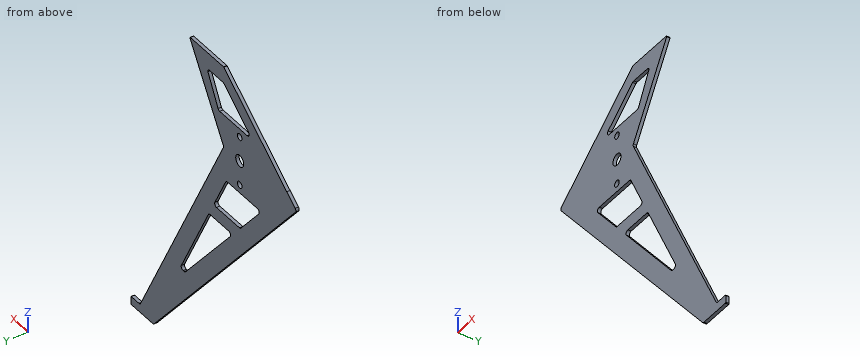
from build123d import *

# Parameters (mm, degrees)
F0_R     = 1.27
F0_R_2   = 2.2225
F1_DEPTH = 1.27


with BuildPart() as f1:
    # F0 (on Front) → F1 (new body)
    with BuildSketch(Plane.XZ):
        with BuildLine():
            Line((14.791388, 63.5), (-3.722544, 63.5))
            ThreePointArc((-3.722544, 63.5), (-3.805236, 63.486163), (-3.878918, 63.446158))
            Line((-3.878918, 63.446158), (-38.962514, 36.037098))
            Line((-38.962514, 36.037098), (-43.621762, 32.397061))
            ThreePointArc((-43.621762, 32.397061), (-44.006646, 31.703164), (-43.775246, 30.944163))
            Line((-43.775246, 30.944163), (-41.186804, 27.852871))
            Line((-41.186804, 27.852871), (35.001432, -63.136264))
            ThreePointArc((35.001432, -63.136264), (35.350553, -63.404586), (35.78041, -63.5))
            Line((35.78041, -63.5), (44.45, -63.5))
            Line((44.45, -63.5), (47.752, -63.5))
            ThreePointArc((47.752, -63.5), (47.931605, -63.425605), (48.006, -63.246))
            Line((48.006, -63.246), (48.006, -60.579))
            ThreePointArc((48.006, -60.579), (47.931605, -60.399395), (47.752, -60.325))
            Line((47.752, -60.325), (43.465528, -60.325))
            ThreePointArc((43.465528, -60.325), (42.933685, -60.174679), (42.559219, -59.768196))
            Line((42.559219, -59.768196), (-3.556335, 31.249344))
            ThreePointArc((-3.556335, 31.249344), (-3.665378, 31.744831), (-3.521239, 32.231268))
            Line((-3.521239, 32.231268), (15.009191, 63.115318))
            ThreePointArc((15.009191, 63.115318), (15.012418, 63.371145), (14.791388, 63.5))
        make_face()
        with BuildLine():
            Line((18.907663, -31.75), (18.272293, -31.75))
            ThreePointArc((18.272293, -31.75), (17.842435, -31.654586), (17.493315, -31.386264))
            Line((17.493315, -31.386264), (-7.390557, -1.668264))
            ThreePointArc((-7.390557, -1.668264), (-7.532165, -0.586142), (-6.611579, 0))
            Line((-6.611579, 0), (3.850543, 0))
            ThreePointArc((3.850543, 0), (4.382385, -0.150321), (4.756851, -0.556804))
            Line((4.756851, -0.556804), (19.813971, -30.274804))
            ThreePointArc((19.813971, -30.274804), (19.773342, -31.265842), (18.907663, -31.75))
        make_face(mode=Mode.SUBTRACT)
        with BuildLine():
            ThreePointArc((-5.801457, 19.05), (-5.269615, 18.899679), (-4.895149, 18.493196))
            Line((-4.895149, 18.493196), (1.153438, 6.555196))
            ThreePointArc((1.153438, 6.555196), (1.112808, 5.564158), (0.24713, 5.08))
            Line((0.24713, 5.08), (-12.566694, 5.08))
            ThreePointArc((-12.566694, 5.08), (-12.996552, 5.175414), (-13.345672, 5.443736))
            Line((-13.345672, 5.443736), (-23.341757, 17.381736))
            ThreePointArc((-23.341757, 17.381736), (-23.483365, 18.463858), (-22.562779, 19.05))
            Line((-22.562779, 19.05), (-5.801457, 19.05))
        make_face(mode=Mode.SUBTRACT)
        with Locations((-12.727872, 22.225)):
            Circle(F0_R, mode=Mode.SUBTRACT)
        with Locations((-12.7, 31.75)):
            Circle(F0_R_2, mode=Mode.SUBTRACT)
        with Locations((-12.7, 41.275)):
            Circle(F0_R, mode=Mode.SUBTRACT)
        with BuildLine():
            ThreePointArc((-3.962149, 56.934633), (-3.667421, 57.094651), (-3.336654, 57.15))
            Line((-3.336654, 57.15), (4.325205, 57.15))
            ThreePointArc((4.325205, 57.15), (4.975285, 56.785541), (5.003509, 56.040801))
            Line((5.003509, 56.040801), (-0.646303, 45.003068))
            ThreePointArc((-0.646303, 45.003068), (-1.020653, 44.599226), (-1.550708, 44.45))
            Line((-1.550708, 44.45), (-16.991694, 44.45))
            ThreePointArc((-16.991694, 44.45), (-17.952345, 45.135233), (-17.617189, 46.266633))
            Line((-17.617189, 46.266633), (-3.962149, 56.934633))
        make_face(mode=Mode.SUBTRACT)
    extrude(amount=F1_DEPTH)


solid = f1.part
Check sheet for the modelled part. Datum: model origin and axes. Units: mm. Coordinates: 2 decimals unless noted, no trailing zeros. Write each loop counter-clockwise with the first axis right and the second up, starting at its lowest first coordinate (ties: lowest second). Pieces come first, ordered by that corner, then holes. Notation, with made-up numbers: M 46,39 L 88,39 A17 ccw 88,65 Z; hole C -16.75,-22 d5. An arc over 180 degrees is marked long. Answer as CSV lines item,"result".
Q1. Cross-section at C-C (y = -0.2). Count the separate pieces of the cut face and the enclosed holes in it, then the cut area to 3 significant figures.
Check result:
separate pieces,"1"
enclosed holes,"6"
area,"2,640 mm^2"
Q2. Cross-section at D-D (z = -48). Record the boundary of the cut face in (x, y), then the cut area to 3 significant figures.
Check result:
outline,"M 22.33,-1.27 L 36.6,-1.27 L 36.6,0 L 22.33,0 Z"
area,"18.1 mm^2"
Q3. Cross-section at B-B (x = 7). Record the boundary of the cut face in (y, z).
Check result:
outline,"M -1.27,-29.7 L 0,-29.7 L 0,-18.85 L -1.27,-18.85 Z; M -1.27,-4.98 L 0,-4.98 L 0,10.41 L -1.27,10.41 Z; M -1.27,49.77 L 0,49.77 L 0,63.5 L -1.27,63.5 Z"
Q4. Cross-section at A-A (z = -16.5). Record the boundary of the cut face in (x, y).
Check result:
outline,"M -4.05,-1.27 L 5.03,-1.27 L 5.03,0 L -4.05,0 Z; M 12.83,-1.27 L 20.64,-1.27 L 20.64,0 L 12.83,0 Z"
Q5. Material ranges on probe 1 along Z at (x, y) = (-10, -0.05); probe 2 along X at (y, z) = (-1.1, 31.5); probe 3 along Z at (x, y) = (0, -1.1), recorded low to high. Write a range as from..to.
Check result:
probe 1,"-9.39..5.08, 19.05..44.45, 52.22..58.66"
probe 2,"-44.01..-14.91, -10.49..-3.64"
probe 3,"-21.34..-10.49, 0..5.08, 8.83..24.23, 38.1..46.27, 57.15..63.5"
Q6. Go/stop test with flat-tipped pins: pin 1 (0.6 mm diameter, centred on x = 0.5, y = -1, fed in from -Z); pin 2 (0.6 mm diameter, centred on x = -0.5, y = -0.5, fed in from -Z); pin 3 (0.6 mm diameter, centred on x = 46, y = -1, fed in from +Z) (3 decimals); pin 4 (3.5 mm diameter, centred on x = -12.7, z = 31.75, fed in from -Y). Record where each tip stops, or that it passes through.
Check result:
pin 1,"z = -22.29"
pin 2,"z = -21.1"
pin 3,"z = -60.325"
pin 4,"through"
